```python
from build123d import *

# Parameters (mm, degrees)
SKETCH1_W             = 100
SKETCH1_H             = 10
BOSS_EXTRUDE1_DEPTH   = 3
FILLET1_R             = 3
F_3_0MM_DOWEL_HOLE1_D = 3
SKETCH2_W             = 47
SKETCH2_H             = 0.1
CUT_EXTRUDE1_DEPTH    = 10


with BuildPart() as part:
    # Sketch1 → Boss-Extrude1 (new body)
    with BuildSketch(Plane(origin=(0, 0, 0), x_dir=(1, 0, 0), z_dir=(0, 1, 0))):
        Rectangle(SKETCH1_W, SKETCH1_H)
    extrude(amount=BOSS_EXTRUDE1_DEPTH)

    # Fillet1
    fillet1_edges = [part.edges().sort_by_distance(p)[0] for p in [
        (50, 1.5, 5),
        (-50, 1.5, 5),
        (-50, 1.5, -5),
        (50, 1.5, -5),
    ]]
    fillet(fillet1_edges, radius=FILLET1_R)

    # Ø3.0mm Dowel Hole1 (through all)
    with Locations(Plane(origin=(0, 3, 0), x_dir=(1, 0, 0), z_dir=(0, 1, 0))):
        with Locations((46, 0), (6, 0)):
            Hole(F_3_0MM_DOWEL_HOLE1_D / 2)

    # Sketch2 → Cut-Extrude1 (cut)
    with BuildSketch(Plane(origin=(0, 3, 0), x_dir=(1, 0, 0), z_dir=(0, 1, 0))):
        with Locations((-26.5, 0)):
            Rectangle(SKETCH2_W, SKETCH2_H)
    extrude(amount=-CUT_EXTRUDE1_DEPTH, mode=Mode.SUBTRACT)


solid = part.part
```
Verification items for the finished model (mm, model axes). Coordinates: 2 decimals unless noted, no trailing zeros. Order: outer loops, then holes, each group sorted by start corner. A loop starts at its lowest first (then second) coordinate and runs counter-clockwise, first axis right, second up. Notation, with made-up numbers: (88.5, 61) -> (131.5, 61) arc R20 cw to (131.5, 72) -> close; hole circle Ø9 at (10, 29). An arc over 180 degrees is marked (long way). Answer as CSV lines item,"result". Start each with the question number.
1) Cross-section at C-C, the plane z = -4. Record the boundary of the cut face in (x, y), then the cut area to 3 significant figures.
2) Material ranges on L1, parallel to X at y = 1, z = 1.25; L2, parallel to X at y = 1.6, z = 0.5; L3, parallel to Z at x = 46, y = 1.55, recorded low to high. Write a range as [from, to].
3) Release check for a two-part mould opening along Z. For faces 1 (the face through (-49.14, 1.52, 4.1)), 2 (the face through (-1, 3, 0)), 3 (the face through (7.2, 1.5, 0.9)) record: released by +Z, released by -Z, zero draft, split by the parting line, or undercut.
4) Cross-section at B-B, the plane x = 46. Record the boundary of the cut face in (y, z).
5) Cross-section at A-A, the plane y = 0.95. Record the boundary of the cut face in (x, z), then the cut area to 3 significant figures.
6) Gauge pin test, flat end, axial feed: pin 1 Ø1 at (y, z) = (2, -3) entering from +X. Record the tip position at first contact, or that the pin passes through.
Conclusion:
1,outline,"(-49.24, 0) -> (49.24, 0) -> (49.24, 3) -> (-49.24, 3) -> close"
1,area,"295 mm²"
2,L1,"x = [-50, 5.17], [6.83, 45.17], [46.83, 50]"
2,L2,"x = [-50, 4.59], [7.41, 44.59], [47.41, 50]"
2,L3,"z = [-5, -1.5], [1.5, 5]"
3,face 1,"released by +Z"
3,face 2,"zero draft"
3,face 3,"undercut"
4,outline,"(0, -5) -> (3, -5) -> (3, -1.5) -> (0, -1.5) -> close; (0, 1.5) -> (3, 1.5) -> (3, 5) -> (0, 5) -> close"
5,outline,"(-50, -2) arc R3 ccw to (-47, -5) -> (47, -5) arc R3 ccw to (50, -2) -> (50, 2) arc R3 ccw to (47, 5) -> (-47, 5) arc R3 ccw to (-50, 2) -> (-50, 0.05) -> (-3, 0.05) -> (-3, -0.05) -> (-50, -0.05) -> close; hole circle Ø3 at (6, 0); hole circle Ø3 at (46, 0)"
5,area,"973 mm²"
6,pin 1,"stops at x = 49.96"
